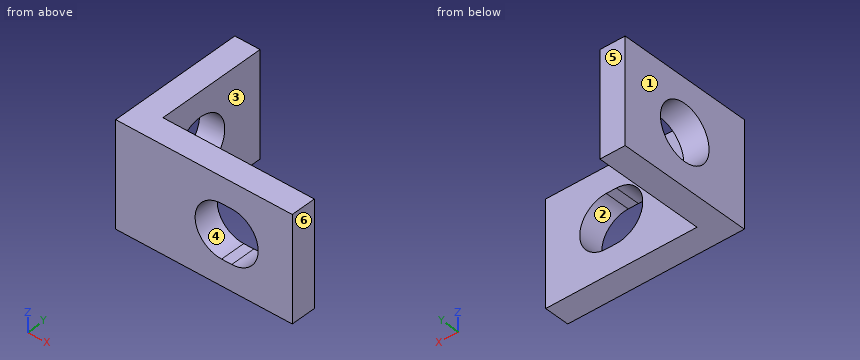
```python
from build123d import *

# Parameters (mm, degrees)
EXTRUDE_1_DEPTH     = 4.14
SKETCH_3_R          = 1.1
CUT_EXTRUDE_1_DEPTH = 10.762151402
CUT_EXTRUDE_2_DEPTH = 10.762151402


with BuildPart() as part:
    # 草图1 → 凸台-拉伸1 (new body)
    with BuildSketch(Plane.XY):
        Polygon((0, 0), (0, 5.4), (1, 5.4), (1, 1), (7, 1), (7, 0), align=None)
    extrude(amount=EXTRUDE_1_DEPTH)

    # 草图3 → 切除-拉伸1 (cut, through all)
    with BuildSketch(Plane.ZY):
        with Locations((2.07, 2.7)):
            Circle(SKETCH_3_R)
    extrude(amount=-CUT_EXTRUDE_1_DEPTH, mode=Mode.SUBTRACT)

    # 草图4 → 切除-拉伸2 (cut, through all)
    with BuildSketch(Plane.XZ):
        with BuildLine():
            Line((4.6, 1.02), (4.2, 1.02))
            ThreePointArc((4.2, 1.02), (3.15, 2.07), (4.2, 3.12))
            Line((4.2, 3.12), (4.6, 3.12))
            ThreePointArc((4.6, 3.12), (5.65, 2.07), (4.6, 1.02))
        make_face()
    extrude(amount=-CUT_EXTRUDE_2_DEPTH, mode=Mode.SUBTRACT)


solid = part.part
```
Geometry: final body of the model. Coordinates: model frame, mm. Face numbers are marked on the shaded views. A direction names the side the tool comes from. Coordinates: 2 decimals unless noted, no trailing zeros. Order: outer loops, then holes, each group sorted by start corner. A loop starts at its lowest first (then second) coordinate and runs counter-clockwise, first axis right, second up. Notation, with made-up numbers: (47, 65.25) - (92, 65.25) arc R29 cw to (92, 85.25) - close; hole circle Ø10 at (-12.75, 29.25). An arc over 180 degrees is marked (long way). Write each question's results on one line, items separated by ' | '.
(1) First-contact query: pin 1 Ø1.2 at (x, z) = (3, 2) entering from +Y; pin 2 Ø1.5 at (y, z) = (3.5, 0.5) entering from +X. Flat tips, straight axial feed; report the tip coordinate or a pass-through.
Values found:
pin 1: stops at y = 1 | pin 2: stops at x = 1
(2) Section query B-B, the plane z = 2.07. Return the cut outline in (x, y).
Values found:
outline: (0, 0) - (3.15, 0) - (3.15, 1) - (1, 1) - (1, 1.6) - (0, 1.6) - close; (0, 3.8) - (1, 3.8) - (1, 5.4) - (0, 5.4) - close; (5.65, 0) - (7, 0) - (7, 1) - (5.65, 1) - close
(3) Set-up query: the marked faces 1, 2 and 3. Return all of +Z, -Z, +X, -X, +Y, -Y with unobstructed straight access to the full face (end or side cutting, diameter ignored); none if empty.
Values found:
face 1: +Z, -Z, -X, +Y, -Y | face 2: +Y, -Y | face 3: +Z, -Z, +X, +Y
(4) Mould query, pull axis X, two halves, no side actions, for the marked faces 4, 5 and 6. Classes: +X half, -X half, draft (parallel to the pull), parting line (faces both ways), or undercut.
Values found:
face 4: undercut | face 5: draft | face 6: +X half
(5) Section query D-D, the plane x = 1.5. Return the cut outline in (y, z).
Values found:
outline: (0, 0) - (1, 0) - (1, 4.14) - (0, 4.14) - close
(6) Section query A-A, the plane x = 4.5. Return the cut outline in (y, z), plus the area to 3 significant figures.
Values found:
outline: (0, 0) - (1, 0) - (1, 1.02) - (0, 1.02) - close; (0, 3.12) - (1, 3.12) - (1, 4.14) - (0, 4.14) - close | area: 2.04 mm²
(7) Section query C-C, the plane y = 2.7. Return the cut outline in (x, z), plus the area to 3 significant figures.
Values found:
outline: (0, 0) - (1, 0) - (1, 0.97) - (0, 0.97) - close; (0, 3.17) - (1, 3.17) - (1, 4.14) - (0, 4.14) - close | area: 1.94 mm²
(8) Line query: line 1 (Y direction, x = 0.7, z = 2.07); line 2 (X direction, y = 4.3, z = 0.35); line 3 (Z direction, x = 5.5, y = 0.55). Output: solid intervals per line, ascending. Write a range as [from, to].
Values found:
line 1: y = [0, 1.6], [3.8, 5.4] | line 2: x = [0, 1] | line 3: z = [0, 1.53], [2.61, 4.14]
